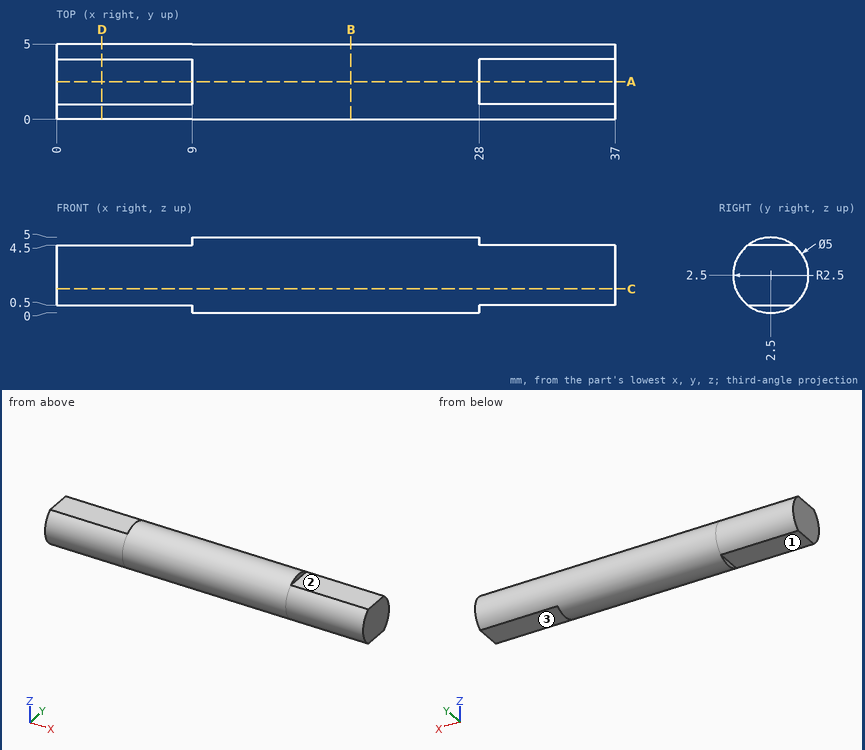
Geometry check sheet. Reference: drawing and pictorial views, mm from the part's lowest x, y, z. A direction names the side the tool comes from. Coordinates: 2 decimals unless noted, no trailing zeros. Order: outer loops, then holes, each group sorted by start corner. A loop starts at its lowest first (then second) coordinate and runs counter-clockwise, first axis right, second up.
Item 1: Section check C-C (z = 1.6). Enter the section's corners in (x, y), plus the area to 3 significant figures.
Item 2: Depth check by flat-ended pin: pin 1 (1.5 mm diameter, centred on y = 3, z = 0.5, fed in from -X); pin 2 (0.9 mm diameter, centred on x = 31.5, y = 2, fed in from -Z); pin 3 (0.6 mm diameter, centred on y = 2, z = 0, fed in from +X); pin 4 (1.5 mm diameter, centred on x = 29, z = 1, fed in from +Y). Enter the tip coordinate at first touch or a pass-through.
Item 3: Scan lines: line 1 along Z through (x, y) = (8, 3.2); line 2 along Z through (x, y) = (30.5, 4.5); line 3 along X through (y, z) = (2.95, 4.6). Record each from-to range of solid material in increasing order.
Item 4: Section check B-B (x = 19.5). Enter the section's corners in (y, z), plus the area to 3 significant figures.
Item 5: Section check D-D (x = 3). Enter the section's corners in (y, z), plus the area to 3 significant figures.
Item 6: Section check A-A (y = 2.5). Enter the section's corners in (x, z), plus the area to 3 significant figures.
Item 7: Tool access check on the marked faces 1, 2 and 3. Record the directions out of +Z, -Z, +X, -X, +Y, -Y that give a thin tool (end or side, any length) a straight path to the whole face; none if there is none.
Check sheet entries:
1. outline: (0, 0.17) - (37, 0.17) - (37, 4.83) - (0, 4.83) - close
1. area: 173 mm2
2. pin 1: stops at x = 0
2. pin 2: stops at z = 0.5
2. pin 3: stops at x = 28
2. pin 4: stops at y = 4.88
3. line 1: z = 0.5 to 4.5
3. line 2: z = 1 to 4
3. line 3: x = 9 to 28
4. outline: circle Ø5 at (2.5, 2.5)
4. area: 19.6 mm2
5. outline: (1, 0.5) - (4, 0.5) arc R2.5 ccw to (4, 4.5) - (1, 4.5) arc R2.5 ccw to start
5. area: 17.6 mm2
6. outline: (0, 0.5) - (9, 0.5) - (9, 0) - (28, 0) - (28, 0.5) - (37, 0.5) - (37, 4.5) - (28, 4.5) - (28, 5) - (9, 5) - (9, 4.5) - (0, 4.5) - close
6. area: 167 mm2
7. face 1: -Z, -X, +Y, -Y
7. face 2: +Z, +X, +Y, -Y
7. face 3: -Z, +X, +Y, -Y
